from build123d import *

# Parameters (mm, degrees)
SKETCH_1_W           = 62
SKETCH_1_H           = 100
F_5_PCB_100X62_DEPTH = 1.6
EXTRUDE_START        = 1.6
SKETCH_2_W           = 16
SKETCH_2_H           = 21
EXTRUDE_312_DEPTH    = 16
USB_START            = 1.6
SKETCH_3_W           = 26
SKETCH_3_H           = 15
USB_DEPTH            = 14
SKETCH_4_W           = 12
SKETCH_4_H           = 17
EXTRUDE_463_DEPTH    = 6
SKETCH_5_W           = 38
SKETCH_5_H           = 38
EXTRUDE_553_DEPTH    = 15


with BuildPart() as part:
    # 草图1 → 香橙派5_PCB官方外形100x62 (new body)
    with BuildSketch(Plane.XY):
        Rectangle(SKETCH_1_W, SKETCH_1_H)
    extrude(amount=F_5_PCB_100X62_DEPTH)

    # 草图2 → Extrude 312 (add)
    with BuildSketch(Plane.XY.offset(EXTRUDE_START)):
        with Locations((19, -43)):
            Rectangle(SKETCH_2_W, SKETCH_2_H)
    extrude(amount=EXTRUDE_312_DEPTH)

    # 草图3 → USB插拔包络_需按实物替换 (add)
    with BuildSketch(Plane.XY.offset(USB_START)):
        with Locations((-13, -43)):
            Rectangle(SKETCH_3_W, SKETCH_3_H)
    extrude(amount=USB_DEPTH)

    # 草图4 → Extrude 463 (add)
    with BuildSketch(Plane.XY.offset(EXTRUDE_START)):
        with Locations((-25, 27)):
            Rectangle(SKETCH_4_W, SKETCH_4_H)
    extrude(amount=EXTRUDE_463_DEPTH)

    # 草图5 → Extrude 553 (add)
    with BuildSketch(Plane.XY.offset(EXTRUDE_START)):
        with Locations((1, 8)):
            Rectangle(SKETCH_5_W, SKETCH_5_H)
    extrude(amount=EXTRUDE_553_DEPTH)


solid = part.part
Can you work these out from the model? Positions are in its coordinate system, mm. A direction names the side the tool comes from. Round coordinates to 2 decimals unless told otherwise and drop trailing zeros. Write each loop counter-clockwise with the first axis right and the second up, starting at its lowest first coordinate (ties: lowest second). Pieces come first, ordered by that corner, then holes. Notation, with made-up numbers: (14.25, 64.5) -> (27.25, 64.5) arc R31 ccw to (27.25, 92.5) -> close; hole circle Ø1 at (56, -24). An arc over 180 degrees is marked (long way). Use one line per item in the form item = value. Start each with the question number.
Q1. If I drill on probe 1 along Y at (x, z) = (19, 6); probe 2 along X at (y, z) = (-40, 15); probe 3 along Y at (x, z) = (-6, 6), over which ranges is the centre line in solid material (lowest first)? Write a range as [from, to].
Q2. Which directions (+Z, -Z, +X, -X, +Y, -Y) give clear straight access to the entire face, cutting with the end or side of a thin tool? Please do faces 1 (the face through (-25, 18.5, 5)), 2 (the face through (1, 8, 16.6)), 3 (the face through (-25, 27, 7.6)), 4 (the face through (19, -52, 1.6)), 5 (the face through (1, 27, 9)).
Q3. Imagine slicing it at D-D (y = 6). Please give me the cut outline in (x, z), then the cut area to 3 significant figures.
Q4. We'd pull the mould along Y, two halves only. Please class faces 6 (the face through (-19, 27, 5)), 7 (the face through (-13, -50.5, 9)), 8 (the face through (1, -11, 9)): +Y half, -Y half, draft (parallel to the pull), parting line (faces both ways), or undercut.
Q5. Imagine slicing it at A-A (z = 4). Please give me the cut outline in (x, y).
Q6. Imagine slicing it at B-B (z = 10). Please give me the cut outline in (x, y).
Q7. I'm going to push flat-ended pins straight in: P1, Ø7.5, axis at x = 8, z = 8.5, coming from the -Y side; P2, Ø5, axis at x = -4.5, y = -7.5, coming from the +Z side; P3, Ø5, axis at x = -25, z = 5.5, coming from the -Y side; P4, Ø7.5, axis at x = -10.5, y = -45.5, coming from the +Z side. Where does each tip first touch, or does it pass through?
Q8. Imagine slicing it at C-C (x = -9). Please give me the cut outline in (y, z).
Worked out:
q1.probe_1 = [-53.5, -32.5], [-11, 27]
q1.probe_2 = [-26, 0], [11, 27]
q1.probe_3 = [-50.5, -35.5], [-11, 27]
q2.face_1 = +Z, -X
q2.face_2 = +Z, +X, -X, +Y
q2.face_3 = +Z, -X, +Y
q2.face_4 = -Z, +X, -X, -Y
q2.face_5 = +Z, +X, +Y
q3.outline = (-31, 0) -> (31, 0) -> (31, 1.6) -> (20, 1.6) -> (20, 16.6) -> (-18, 16.6) -> (-18, 1.6) -> (-31, 1.6) -> close
q3.area = 669 mm^2
q4.face_6 = draft
q4.face_7 = -Y half
q4.face_8 = undercut
q5.outline = (-31, 18.5) -> (-19, 18.5) -> (-19, 35.5) -> (-31, 35.5) -> close; (-26, -50.5) -> (0, -50.5) -> (0, -35.5) -> (-26, -35.5) -> close; (-18, -11) -> (20, -11) -> (20, 27) -> (-18, 27) -> close; (11, -53.5) -> (27, -53.5) -> (27, -32.5) -> (11, -32.5) -> close
q6.outline = (-26, -50.5) -> (0, -50.5) -> (0, -35.5) -> (-26, -35.5) -> close; (-18, -11) -> (20, -11) -> (20, 27) -> (-18, 27) -> close; (11, -53.5) -> (27, -53.5) -> (27, -32.5) -> (11, -32.5) -> close
q7.P1 = -53.5
q7.P2 = 16.6
q7.P3 = -50.5
q7.P4 = 15.6
q8.outline = (-50.5, 1.6) -> (-50, 1.6) -> (-50, 0) -> (50, 0) -> (50, 1.6) -> (27, 1.6) -> (27, 16.6) -> (-11, 16.6) -> (-11, 1.6) -> (-35.5, 1.6) -> (-35.5, 15.6) -> (-50.5, 15.6) -> close
